Source: CAD feature listing. Evaluate the final solid. Frame: model axes, mm. Face numbers are marked on the shaded views. Coordinates: 2 decimals unless noted, no trailing zeros. Write each loop counter-clockwise with the first axis right and the second up, starting at its lowest first coordinate (ties: lowest second). Pieces come first, ordered by that corner, then holes. Notation, with made-up numbers: M 7,88 L 60,88 A24 cw 60,122 Z; hole C 6,62.5 d5. An arc over 180 degrees is marked long. One line per item, written item: value. Start each with the question number.
Item 1: Pin query (flat end, axial travel): P1, Ø1.5, axis at x = -1, z = -8.5, coming from the +Y side. Return the tip coordinate at first contact, or that it passes through.
Item 2: Ray query, L1, parallel to Y at x = 0, z = -3.25; L2, parallel to Y at x = -0.35, z = 16; L3, parallel to Z at x = 1.45, y = 1.65. Return the intervals inside material, ascending. Write a range as from..to.
Item 3: Mould query, pull axis Y, two halves, no side actions, for the marked faces 1 and 2. Classes: released by +Y, released by -Y, zero draft, split by the parting line, or undercut.
Item 4: Cut plane A-A, the plane x = 0. Output: boundary loops of the cut face in (y, z).
Item 5: Cut plane C-C, the plane z = 0. Output: boundary loops of the cut face in (x, y), then the cut area to 3 significant figures.
Autodesk Inventor part; units mm, degrees
ref_plane "YZ Plane" through (0, 0, 0) normal (1, 0, 0) x (0, 1, 0)
ref_plane "XZ Plane" through (0, 0, 0) normal (0, 1, 0) x (-1, 0, 0)
ref_plane "XY Plane" through (0, 0, 0) normal (0, 0, 1) x (1, 0, 0)
sketch "Sketch1" plane through (0, 0, 0) normal (0, 0, 1) x (1, 0, 0)
  circle A0 centre (0, 0) radius 3
  circle A1 centre (0, 0) radius 2
  dimension "d0" = 6
  dimension "d1" = 4
extrude "Extrusion1" add sketch "Sketch1" along normal mid plane 30
sketch "Sketch2" plane through (0, 0, 0) normal (1, 0, 0) x (0, 1, 0)
  line L0 (3, 15) -> (-3, 15) construction
  line L1 (0, 15) -> (0, 19) construction
  line L2 (-3, -15) -> (-3, 15) construction
  line L3 (-3, 15) -> (-1, 19)
  line L4 (-1, 19) -> (-0.5, 19)
  line L5 (-0.5, 19) -> (-2.5, 15)
  line L6 (-3, 15) -> (-2.5, 15)
  point P0 (0, 0)
  point P1 (-0.75, 19)
  dimension "d4" = 4
  dimension "d9" = 2
  dimension "d10" = 1
revolve "Revolution1" add sketch "Sketch2" angle 360 about axis through (0, 0, 15) along (0, 0, 1)
properties part number "Nozzle"
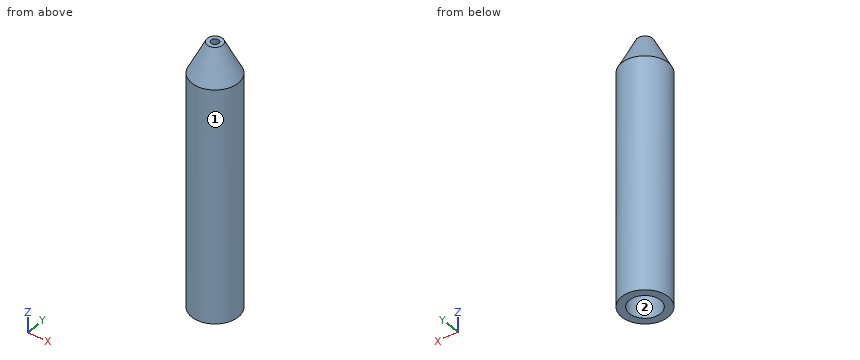
From the geometry:
1. P1: stops at y = 2.99
2. L1: y = -3..-2, 2..3
2. L2: y = -2.48..-1.97, 1.97..2.48
2. L3: z = -15..15, 15.61..16.61
3. face 1: split by the parting line
3. face 2: undercut
4. outline: M -3,-15 L -2,-15 L -2,15 L -2.5,15 L -0.5,19 L -1,19 L -3,15 Z; M 0.5,19 L 2.5,15 L 2,15 L 2,-15 L 3,-15 L 3,15 L 1,19 Z
5. outline: C 0,0 d6; hole C 0,0 d4
5. area: 15.7 mm²
